Could you check a few things on this model? Use its own coordinates, in mm. Face numbers are marked on the shaded views. Round coordinates to 2 decimals unless told otherwise and drop trailing zeros. Loops run counter-clockwise (first coordinate to the right, second up) from the corner with the lowest first, then second, coordinate; pieces in that order, holes last. Notation, with made-up numbers: (-28, 44) -> (29, 44) arc R23 cw to (29, 53) -> close; hole circle Ø8 at (76, -14.5). An arc over 180 degrees is marked (long way). One line per item, written item: value.
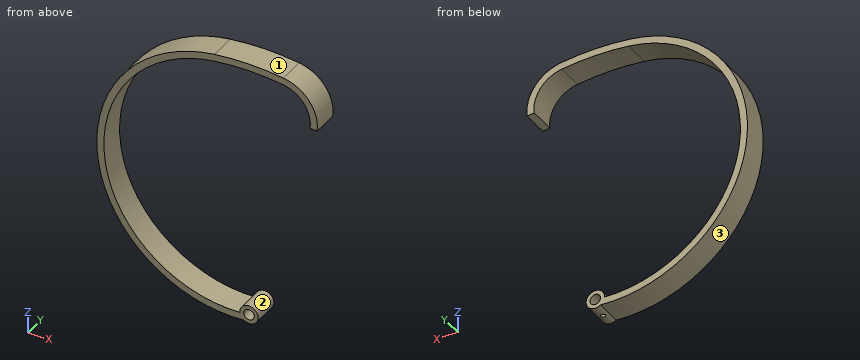
```python
from build123d import *

# Parameters (mm, degrees)
ESQUISSE1_R        = 3
BOSS_EXTRU_3_DEPTH = 15
ESQUISSE7_W        = 1.25
ESQUISSE7_H        = 5.244372399


with BuildPart() as part:
    # Esquisse1 → Boss.-Extru.3 (new body)
    with BuildSketch(Plane(origin=(0, 0, 0), x_dir=(1, 0, 0), z_dir=(0, 1, 0))):
        with BuildLine():
            Line((34.729410673, -124.285932568), (38.695354514, -123.765078027))
            ThreePointArc((38.695354514, -123.765078027), (34.282632836, -140.212837317), (19.532045284, -148.722894024))
            ThreePointArc((19.532045284, -148.722894024), (-0.023643562, -149.999998137), (-19.578928833, -148.716729206))
            ThreePointArc((-19.578928833, -148.716729206), (-86.077469284, -64.054307062), (-2.940851082, 4.342215653))
            ThreePointArc((-2.940851082, 4.342215653), (4.510953097, -2.674835324), (-5.220739084, 0.49731808))
            ThreePointArc((-5.220739084, 0.49731808), (-82.19944379, -65.452964988), (-19.056824064, -144.750949761))
            ThreePointArc((-19.056824064, -144.750949761), (-0.023013067, -145.999998186), (19.011190743, -144.756950184))
            ThreePointArc((19.011190743, -144.756950184), (31.109987274, -137.776791312), (34.729410673, -124.285932568))
        make_face()
        with Locations(Location((0, 0, 0), (0, 0, 270))):
            Circle(ESQUISSE1_R, mode=Mode.SUBTRACT)
    extrude(amount=BOSS_EXTRU_3_DEPTH)

    # Esquisse7 → Trou taraudé M3x0.51 (revolve, cut)
    with BuildSketch(Plane(origin=(0, 7.5, 0), x_dir=(0, -1, 0), z_dir=(1, 0, 0))):
        with Locations((0.625, 2.6221862)):
            Rectangle(ESQUISSE7_W, ESQUISSE7_H)
    revolve(axis=Axis((0, 7.5, 6.35), (0, 0, -1)), mode=Mode.SUBTRACT)


solid = part.part
```
(1) Imagine slicing it at C-C on z = 106.5. Write out the boundary of the cut face in (x, y), then the cut area to 3 significant figures.
Results below:
outline: (-78.55, 0) -> (-74.06, 0) -> (-74.06, 15) -> (-78.55, 15) -> close
area: 67.4 mm²
(2) Imagine slicing it at A-A on y = 2. Write out the boundary of the cut face in (x, z), then the cut area to 3 significant figures.
Results below:
outline: (-19.58, 148.72) arc R77 ccw to (-2.94, -4.34) arc R5.24 ccw (long way) to (-5.22, -0.5) arc R73 cw to (-19.06, 144.75) arc R146 cw to (19.01, 144.76) arc R18.25 cw to (34.73, 124.29) -> (38.7, 123.77) arc R22.25 ccw to (19.53, 148.72) arc R150 ccw to start; hole circle Ø6 at (0, 0)
area: 1,260 mm²
(3) Please list where these lines run through material, in increasing order: L1, parallel to Z at x = 0, y = 3.5; L2, parallel to Y at x = 0, z = -3.55; L3, parallel to Z at x = -18, y = 3.75.
Results below:
L1: z = -5.24 to -3, 3 to 5.24, 146 to 150
L2: y = 0 to 6.25, 8.75 to 15
L3: z = -4.16 to -0.13, 144.89 to 148.92
(4) Imagine slicing it at B-B on x = 27.5. Write out the boundary of the cut face in (y, z).
Results below:
outline: (0, 141.33) -> (15, 141.33) -> (15, 146.08) -> (0, 146.08) -> close
(5) For pin 1 Ø1.5 at (x, y) = (-6, 5.5) entering from -Z; pin 2 Ø3 at (x, y) = (-54, 4.5) entering from +Z; pin 3 Ø8 at (x, y) = (-41, 4) entering from -Z, each with a flat end and sliding along its axis, tell me the tip position at first contact or that it passes through.
Results below:
pin 1: stops at z = -4.57
pin 2: stops at z = 136.27
pin 3: stops at z = 0.44
(6) We'd pull the mould along Z, two halves only. Please class the marked faces 1, 2 and 3: +Z half, -Z half, draft (parallel to the pull), parting line (faces both ways), or undercut.
Results below:
face 1: +Z half
face 2: undercut
face 3: parting line
